Geometry: final body of the model. Coordinates: model frame, mm. Coordinates: 2 decimals unless noted, no trailing zeros. Write each loop counter-clockwise with the first axis right and the second up, starting at its lowest first coordinate (ties: lowest second). Pieces come first, ordered by that corner, then holes. Notation, with made-up numbers: M 77,52 L 123,52 A18 ccw 123,83 Z; hole C 87.5,-19 d4. An arc over 180 degrees is marked long. Write item = value, one per line. Start each with the question number.
Item 1: Section B-B on x = 17.5. Output: boundary loops of the cut face in (y, z).
Item 2: Ray query, L1, parallel to X at y = 2.5, z = 3.15; L2, parallel to Y at x = 32.5, z = 1.1; L3, parallel to Y at x = 33, z = 3.45. Return the intervals inside material, ascending. Write a range as [from, to].
Item 3: Section C-C on y = 2.5. Output: boundary loops of the cut face in (x, z).
Item 4: Section A-A on z = 1.95. Output: boundary loops of the cut face in (x, y).
Item 5: Section D-D on y = 4.7. Output: boundary loops of the cut face in (x, z), plus the area to 3 significant figures.
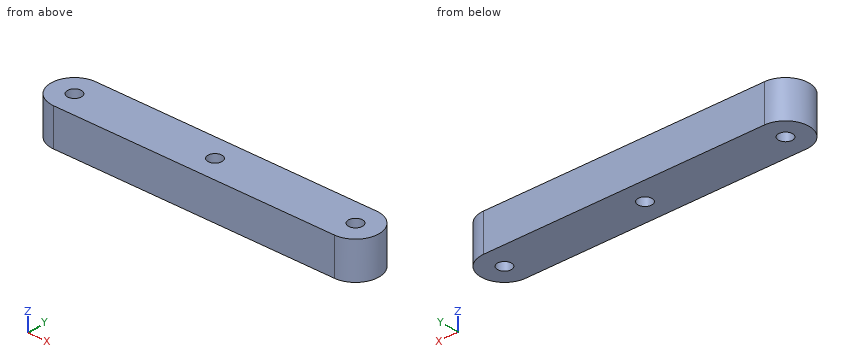
Autodesk Inventor part; units mm, degrees
ref_plane "YZ Plane" through (0, 0, 0) normal (1, 0, 0) x (0, 1, 0)
ref_plane "XZ Plane" through (0, 0, 0) normal (0, 1, 0) x (-1, 0, 0)
ref_plane "XY Plane" through (0, 0, 0) normal (0, 0, 1) x (1, 0, 0)
sketch "Skizze1" plane through (0, 0, 0) normal (0, 0, 1) x (1, 0, 0)
  line L0 (2.5, 0) -> (32.5, 0)
  line L1 (35, 2.5) -> (35, 2.5)
  line L2 (32.5, 5) -> (2.5, 5)
  line L3 (0, 2.5) -> (0, 2.5)
  arc A0 (2.5, 5) -> (0, 2.5) centre (2.5, 2.5) ccw
  arc A1 (0, 2.5) -> (2.5, 0) centre (2.5, 2.5) ccw
  arc A2 (35, 2.5) -> (32.5, 5) centre (32.5, 2.5) ccw
  arc A3 (32.5, 0) -> (35, 2.5) centre (32.5, 2.5) ccw
  point P0 (0, 0)
  point P1 (35, 5)
  point P2 (35, 0)
  point P3 (0, 5)
  dimension "d0" = 35
  dimension "d1" = 5
  dimension "d14" = 2.5
extrude "Extrusion1" add sketch "Skizze1" along normal blind 4
sketch "Skizze2" plane through (0, 0, 4) normal (0, 0, 1) x (1, 0, 0)
  line L0 (0, 0) -> (32.5, 0)
  line L1 (0, 0) -> (2.5, 0)
  line L2 (2.5, 0) -> (0, 0)
  line L3 (2.5, 0) -> (2.5, 2.5)
  circle A0 centre (2.5, 2.5) radius 0.75
  line L4 (35, 0) -> (32.5, 0)
  line L5 (32.5, 0) -> (32.5, 2.5)
  circle A1 centre (32.5, 2.5) radius 0.75
  line L6 (0, 0) -> (17.5, 0)
  line L7 (17.5, 0) -> (17.5, 2.5)
  circle A2 centre (17.5, 2.5) radius 0.75
  dimension "d4" = 2.5
  dimension "d5" = 2.5
  dimension "d6" = 2.5
  dimension "d7" = 1.5
  dimension "d8" = 2.5
  dimension "d9" = 17.5
  dimension "d10" = 1.5
  dimension "d11" = 1.5
  dimension "d15" = 2.5
  dimension "d16" = 2.5
extrude "Extrusion2" cut sketch "Skizze2" against normal blind 5
properties part number "Hebel_KLemme_Hebel"
Responses:
q1.outline = M 0,0 L 1.75,0 L 1.75,4 L 0,4 Z; M 3.25,0 L 5,0 L 5,4 L 3.25,4 Z
q2.L1 = [0, 1.75], [3.25, 16.75], [18.25, 31.75], [33.25, 35]
q2.L2 = [0, 1.75], [3.25, 5]
q2.L3 = [0.05, 1.94], [3.06, 4.95]
q3.outline = M 0,0 L 1.75,0 L 1.75,4 L 0,4 Z; M 3.25,0 L 16.75,0 L 16.75,4 L 3.25,4 Z; M 18.25,0 L 31.75,0 L 31.75,4 L 18.25,4 Z; M 33.25,0 L 35,0 L 35,4 L 33.25,4 Z
q4.outline = M 2.5,0 L 32.5,0 A2.5 ccw 32.5,5 L 2.5,5 A2.5 ccw Z; hole C 2.5,2.5 d1.5; hole C 17.5,2.5 d1.5; hole C 32.5,2.5 d1.5
q5.outline = M 1.31,0 L 33.69,0 L 33.69,4 L 1.31,4 Z
q5.area = 129 mm²
